```python
from build123d import *

# Parameters (mm, degrees)
CUT_EXTRUDE2_START = -24.60625
SKETCH2_W          = 1882.3686
SKETCH2_H          = 12.7
CUT_EXTRUDE2_DEPTH = 63.4619
FILLET1_R          = 3.175
CHAMFER1_SIZE      = 1.524


with BuildPart() as part:
    # Sketch1 → Revolve1 (revolve)
    with BuildSketch(Plane(origin=(0, 0, 0), x_dir=(1, 0, 0), z_dir=(0, 1, 0)), mode=Mode.PRIVATE) as revolve1_sk:
        Polygon((-976.376, 0), (-976.376, 31.73095), (-954.024, 31.73095), (-954.024, 22.0218), (-928.2176, 22.0218), (-928.2176, 31.73095), (928.3446, 31.73095), (928.3446, 22.0218), (954.151, 22.0218), (954.151, 31.73095), (976.376, 31.73095), (976.376, 0), align=None)
    revolve(revolve1_sk.sketch.rotate(Axis((-1001.776, 0, 0), (1, 0, 0)), 180), axis=Axis((-1001.776, 0, 0), (1, 0, 0)))

    # Sketch2 → Cut-Extrude2 (cut)
    with BuildSketch(Plane.XY.offset(CUT_EXTRUDE2_START)):
        with Locations((0.0635, 0)):
            Rectangle(SKETCH2_W, SKETCH2_H)
    extrude(amount=-CUT_EXTRUDE2_DEPTH, mode=Mode.SUBTRACT)

    # Fillet1
    fillet1_edges = [part.edges().sort_by_distance(p)[0] for p in [
        (954.151, 0, -22.0218),
        (928.3446, 0, -22.0218),
        (-928.2176, 0, -22.0218),
        (-954.024, 0, -22.0218),
    ]]
    fillet(fillet1_edges, radius=FILLET1_R)

    # Chamfer1
    chamfer1_edges = [part.edges().sort_by_distance(p)[0] for p in [
        (-976.376, 0, -31.73095),
        (976.376, 0, -31.73095),
    ]]
    chamfer(chamfer1_edges, length=CHAMFER1_SIZE)


solid = part.part
```
Can you work these out from the model? Positions are in its coordinate system, mm. A direction names the side the tool comes from. Round coordinates to 2 decimals unless told otherwise and drop trailing zeros. Loops run counter-clockwise (first coordinate to the right, second up) from the corner with the lowest first, then second, coordinate; pieces in that order, holes last. Notation, with made-up numbers: (-10, 63) -> (37, 63) arc R19 ccw to (37, 91) -> close; hole circle Ø8 at (38, 84.25). An arc over 180 degrees is marked (long way). One line per item, written item: value. Start each with the question number.
1. For pin 1 (2 mm diameter, centred on x = 258.5, z = 9, fed in from -Y); pin 2 (5 mm diameter, centred on x = 170, z = -27.5, fed in from +Y); pin 3 (5 mm diameter, centred on x = -166, z = -29, fed in from -Y), each with a flat end and sliding along its axis, tell me the tip position at first contact or that it passes through.
2. If I drill on probe 1 along X at (y, z) = (-22, 16.5); probe 2 along X at (y, z) = (8, 23); probe 3 along Z at (x, y) = (250.5, -2), over which ranges is the centre line in solid material (lowest first)?
3. For faces 1 (the cylindrical face through (964.646, -9.531, 30.266)), 2 (the flat face through (954.151, -24, -9)), which set-ups out of +Z, -Z, +X, -X, +Y, -Y let a thin tool reach every point of the face, with its end or its side?
4. If we section it at A-A, the plane x = -214: Write out the boundary of the cut face in (y, z), then the cut area to 3 significant figures.
5. If we mould it in two halves opening along X, with no side actions, what happens to faces 3 (the flat face through (-976.376, 0, 0)), 4 (the flat face through (928.345, -14.3, 21.1)), 5 (the cylindrical face through (-964.292, -9.531, 30.266))? For each: pulls with the +X half, pulls with the -X half, needs draft (parallel to the pull), parting line crosses it, or undercut.
Calculated:
1. pin 1: stops at y = -30.71
1. pin 2: stops at y = 19.54
1. pin 3: stops at y = -17.45
2. probe 1: x = -976.38 to -954.02, -928.22 to 928.34, 954.15 to 976.38
2. probe 2: x = -976.38 to -953.91, -928.33 to 928.46, 954.04 to 976.38
2. probe 3: z = -24.61 to 31.67
3. face 1: +X, -X
3. face 2: none
4. outline: (-6.35, -31.09) -> (-6.35, -24.61) -> (6.35, -24.61) -> (6.35, -31.09) arc R31.73 ccw (long way) to start
4. area: 3,080 mm²
5. face 3: pulls with the -X half
5. face 4: undercut
5. face 5: needs draft
